Source: CAD feature listing. Evaluate the final solid. Frame: model axes, mm. Face numbers are marked on the shaded views. A direction names the side the tool comes from. Give positions to 0.01 mm unless a question says otherwise; leave off trailing zeros. Order: outer loops, then holes, each group sorted by start corner. A loop starts at its lowest first (then second) coordinate and runs counter-clockwise, first axis right, second up. Notation, with made-up numbers: M 48,59.25 L 96,59.25 A31 cw 96,90.25 Z; hole C 9.5,51 d5. An arc over 180 degrees is marked long. Use CSV: the item, a comma, the result in double quotes. Start each with the question number.
1. Reachability of the marked faces 1 and 2 from +Z, -Z, +X, -X, +Y, -Y: full face, straight path, thin tool, end or side. Return the list, or none.
2. Line query: line 1 along Z through (x, y) = (-2, 3); line 2 along Z through (x, y) = (0.75, -1.5); line 3 along Z through (x, y) = (-1.75, 0.75). Output: solid intervals per line, ascending. Write a range as [from, to].
3. Section query B-B, the plane z = 8.5. Return the cut outline in (x, y).
4. Pin query (flat end, axial travel): P1, Ø0.6, axis at x = 0, y = -0.5, coming from the -Z side; P2, Ø4, axis at y = -2.5, z = 13, coming from the +X side; P3, Ø5, axis at x = -1, z = 17, coming from the +Y side; P4, Ø1.5, axis at x = -3, z = 12.5, coming from the -Y side. Return the tip coordinate at first contact, or that it passes through.
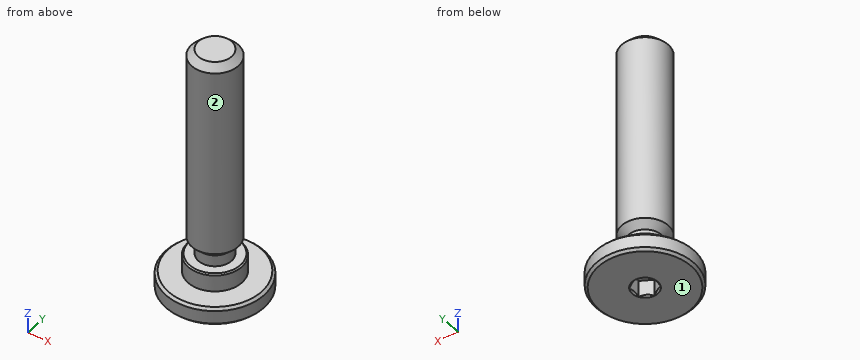
from build123d import *

# Parameters (mm, degrees)
CHAMFER2_SIZE      = 0.5953125
CUT_EXTRUDE1_DEPTH = 1.48828125
CHAMFER1_SIZE      = 0.217805
CHAMFER3_SIZE      = 0.11938


with BuildPart() as part:
    # Sketch13 → Revolve1 (revolve)
    with BuildSketch(Plane(origin=(0, 0, 0), x_dir=(0, 0, -1), z_dir=(1, 0, 0)), mode=Mode.PRIVATE) as revolve1_sk:
        Polygon((1.6002, 4.3561), (0, 4.3561), (0, 2.3876), (-1.6002, 2.3876), (-1.6002, 1.4760575), (-2.6162, 1.4760575), (-3.2115125, 2.07137), (-20.6502, 2.07137), (-20.6502, 0), (1.6002, 0), align=None)
    revolve(revolve1_sk.sketch.rotate(Axis((0, 0, 20.6502), (0, 0, -1)), 180), axis=Axis((0, 0, 20.6502), (0, 0, -1)))

    # Chamfer2
    chamfer2_edges = [part.edges().sort_by_distance(p)[0] for p in [
        (0, 2.07137, 20.6502),
    ]]
    chamfer(chamfer2_edges, length=CHAMFER2_SIZE)

    # Sketch7 → Cut-Extrude1 (cut)
    with BuildSketch(Plane(origin=(0, 0, -1.6002), x_dir=(-1, 0, 0), z_dir=(0, 0, -1))):
        Polygon((0, 1.14567944), (-0.9921875, 0.57283972), (-0.9921875, -0.57283972), (0, -1.14567944), (0.9921875, -0.57283972), (0.9921875, 0.57283972), align=None)
    extrude(amount=-CUT_EXTRUDE1_DEPTH, mode=Mode.SUBTRACT)

    # Chamfer1
    chamfer1_edges = [part.edges().sort_by_distance(p)[0] for p in [
        (0, 4.3561, 0),
        (0, 4.3561, -1.6002),
    ]]
    chamfer(chamfer1_edges, length=CHAMFER1_SIZE)

    # Cut-Extrude2 cone 1 section (on through the dimple's axis) → Cut-Extrude2 (revolve, cut)
    with BuildSketch(Plane(origin=(0, 0, -1.6002), x_dir=(0, 1, 0), z_dir=(1, 0, 0))):
        Polygon((0, 0), (1.14567944, 0), (0, 1.14567944), align=None)
    revolve(axis=Axis((0, 0, -1.6002), (0, 0, 1)), mode=Mode.SUBTRACT)

    # Chamfer3
    chamfer3_edges = [part.edges().sort_by_distance(p)[0] for p in [
        (0, 2.3876, 1.6002),
    ]]
    chamfer(chamfer3_edges, length=CHAMFER3_SIZE)


solid = part.part
Result set:
1,face 1,"-Z, +X, -X, +Y, -Y"
1,face 2,"+Z"
2,line 1,"[-1.6, 0]"
2,line 2,"[-1.6, 1.6], [2.82, 20.45]"
2,line 3,"[-1.6, 1.6], [3.04, 20.22]"
3,outline,"C 0,0 d4.14"
4,P1,"z = -0.11"
4,P2,"x = 2.01"
4,P3,"y = 2.07"
4,P4,"through"
